Design review of the part built by this model. Coordinates are the model's own, in mm. Face numbers are marked on the shaded views. A direction names the side the tool comes from. Give positions to 0.01 mm unless a question says otherwise; leave off trailing zeros. Order: outer loops, then holes, each group sorted by start corner. A loop starts at its lowest first (then second) coordinate and runs counter-clockwise, first axis right, second up. Notation, with made-up numbers: (49.5, 26) -> (66.5, 26) arc R15 ccw to (66.5, 49) -> close; hole circle Ø2 at (-0.5, 31.5). An arc over 180 degrees is marked (long way). One line per item, written item: value. Start each with the question number.
1) Tool access review of the marked faces 1 and 2: name each direction out of +Z, -Z, +X, -X, +Y, -Y from which nothing blocks a thin tool from reaching the whole face with its end or side.
2) Consider section A-A (z = 21). State the section outline as (x, y) points, plus the area to 3 significant figures.
3) Consider section C-C (x = 50). State the section outline as (y, z) points, plus the area to 3 significant figures.
4) Wall thickness on line 1 along X through (y, z) = (33.5, 18); line 2 along Y through (x, z) = (53, 15.5); line 3 along Z through (x, y) = (27, 26.5): over which ranges is each line inside the solid? List them lowest first. Write a range as from..to.
5) The part is to be moulded in two halves that separate along X. For the marked faces 3, 4 and 5, say which applies: released by +X, released by -X, zero draft, split by the parting line, or undercut.
6) Consider section B-B (y = 10.5). State the section outline as (x, z) points, plus the area to 3 significant figures.
7) For pin 1 (14.5 mm diameter, centred on x = 48.5, y = 25.5, fed in from +Z), flat-tipped, find the tip position at first contact; note if it passes through.
from build123d import *

# Parameters (mm, degrees)
F1_DEPTH = 40.64
F3_DEPTH = 38.608


# Not quite as in the source:
# - a feature names something its author has since deleted; it is built from what else it names


with BuildPart() as f1:
    # F0 (on Top) → F1 (new body)
    with BuildSketch(Plane.XY):
        with BuildLine():
            ThreePointArc((0, 2), (0.5857864376, 0.5857864376), (2, 0))
            Line((2, 0), (75.216, 0))
            ThreePointArc((75.216, 0), (76.6302135624, 0.5857864376), (77.216, 2))
            Line((77.216, 2), (77.216, 50.07))
            ThreePointArc((77.216, 50.07), (76.6302135624, 51.4842135624), (75.216, 52.07))
            Line((75.216, 52.07), (2, 52.07))
            ThreePointArc((2, 52.07), (0.5857864376, 51.4842135624), (0, 50.07))
            Line((0, 50.07), (0, 2))
        make_face()
    extrude(amount=F1_DEPTH)

    # F2 (on face) → F3 (cut)
    with BuildSketch(Plane.XY.offset(40.64)):
        with BuildLine():
            Line((74.416, 50.27), (2.8, 50.27))
            ThreePointArc((2.8, 50.27), (2.0928932188, 49.9771067812), (1.8, 49.27))
            Line((1.8, 49.27), (1.8, 2.8))
            ThreePointArc((1.8, 2.8), (2.0928932188, 2.0928932188), (2.8, 1.8))
            Line((2.8, 1.8), (74.416, 1.8))
            ThreePointArc((74.416, 1.8), (75.1231067812, 2.0928932188), (75.416, 2.8))
            Line((75.416, 2.8), (75.416, 49.27))
            ThreePointArc((75.416, 49.27), (75.1231067812, 49.9771067812), (74.416, 50.27))
        make_face()
    extrude(amount=-F3_DEPTH, mode=Mode.SUBTRACT)


solid = f1.part
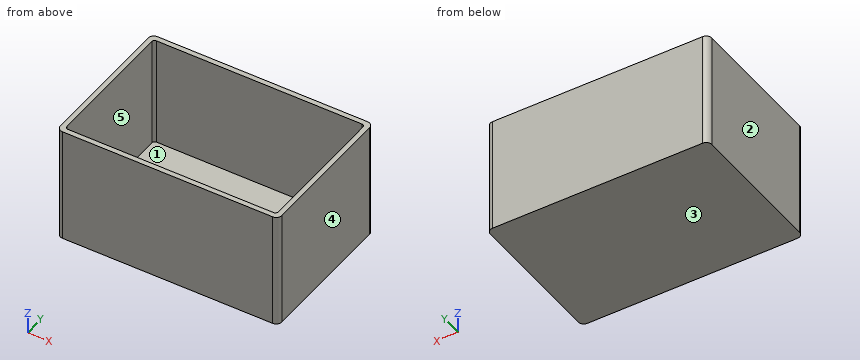
Checked values:
1. face 1: +Z
1. face 2: +Z, -Z, -X, +Y, -Y
2. outline: (0, 2) arc R2 ccw to (2, 0) -> (75.22, 0) arc R2 ccw to (77.22, 2) -> (77.22, 50.07) arc R2 ccw to (75.22, 52.07) -> (2, 52.07) arc R2 ccw to (0, 50.07) -> close; hole (1.8, 2.8) arc R1 ccw to (2.8, 1.8) -> (74.42, 1.8) arc R1 ccw to (75.42, 2.8) -> (75.42, 49.27) arc R1 ccw to (74.42, 50.27) -> (2.8, 50.27) arc R1 ccw to (1.8, 49.27) -> close
2. area: 450 mm^2
3. outline: (0, 0) -> (52.07, 0) -> (52.07, 40.64) -> (50.27, 40.64) -> (50.27, 2.03) -> (1.8, 2.03) -> (1.8, 40.64) -> (0, 40.64) -> close
3. area: 245 mm^2
4. line 1: x = 0..1.8, 75.42..77.22
4. line 2: y = 0..1.8, 50.27..52.07
4. line 3: z = 0..2.03
5. face 3: zero draft
5. face 4: released by +X
5. face 5: undercut
6. outline: (0, 0) -> (77.22, 0) -> (77.22, 40.64) -> (75.42, 40.64) -> (75.42, 2.03) -> (1.8, 2.03) -> (1.8, 40.64) -> (0, 40.64) -> close
6. area: 296 mm^2
7. pin 1: stops at z = 2.03
